The listing builds one solid part. Answer for the finished solid, in the listing's coordinates (mm). Face numbers are marked on the shaded views. A direction names the side the tool comes from. Round coordinates to 2 decimals unless told otherwise and drop trailing zeros. Write each loop counter-clockwise with the first axis right and the second up, starting at its lowest first coordinate (ties: lowest second). Pieces come first, ordered by that corner, then holes.
Item 1: A tool of negligible diameter and unlimited length cuts with its end or side. For the marked faces 4 and 5, from which of +Z, -Z, +X, -X, +Y, -Y can it reach the whole face along a straight path? Write none if from no direction.
Item 2: Each of these flat-tipped pins is pushed along its axis until it touches: pin 1 (6.5 mm diameter, centred on x = 2.83, z = -3.52, fed in from +Y); pin 2 (12 mm diameter, centred on x = -7.5, z = -13, fed in from +Y); pin 3 (6.5 mm diameter, centred on x = 2.5, z = -2.5, fed in from +Y). Where does it stop, or does it pass through?
Item 3: For a pull along Z with two mould halves and no side action, classify the marked faces 1, 2 and 3 as +Z half, -Z half, draft (parallel to the pull), parting line (faces both ways), or undercut.
Item 4: Find section D-D on x = -7.75. Give the vertices of the cut face in (y, z).
Item 5: Find section B-B on x = 0. Give the vertices of the cut face in (y, z).
Item 6: Find section A-A on y = -3.75. Give the vertices of the cut face in (x, z), then the cut area to 3 significant figures.
Item 7: Find section C-C on z = -6.5. Give the vertices of the cut face in (x, y).
Item 8: Find the intervals of material crossed by probe 1 along Y at (x, z) = (14.25, -10); probe 2 along Z at (x, y) = (-10.5, -12); probe 3 along X at (y, z) = (-19.5, 10), in increasing order.
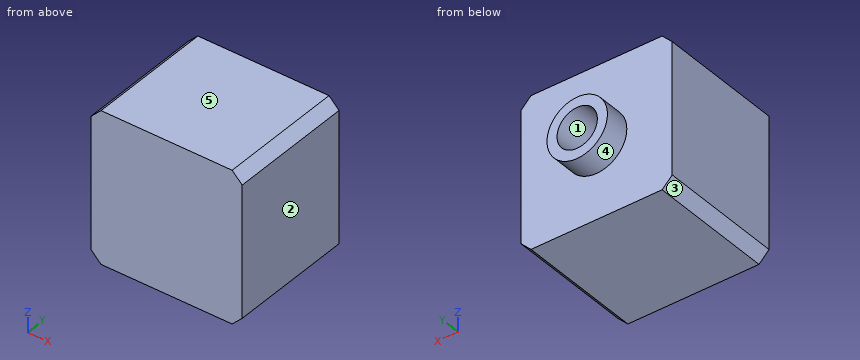
```python
from build123d import *

# Parameters (mm, degrees)
F0_W      = 30
F0_H      = 30
F1_DEPTH  = 25
F3_R      = 6
F4_DEPTH  = 5
F5_SIZE   = 2
F6_SIZE   = 2
F7_SIZE   = 2
F2_R      = 4
F8_DEPTH  = 5
F9_R      = 4
F10_DEPTH = 5


with BuildPart() as f1:
    # F0 (on Front) → F1 (new body)
    with BuildSketch(Plane.XZ):
        with Locations((2.829975, -3.521299)):
            Rectangle(F0_W, F0_H)
    extrude(amount=F1_DEPTH)

    # F3 (on face) → F4 (join)
    with BuildSketch(Plane(origin=(0, 0, 0), x_dir=(-1, 0, 0), z_dir=(0, 1, 0))):
        with Locations((-2.829975, -3.521299)):
            Circle(F3_R)
    extrude(amount=F4_DEPTH)

    # F5
    f5_edges = [f1.edges().sort_by_distance(p)[0] for p in [
        (17.829975, -12.5, 11.478701),
    ]]
    chamfer(f5_edges, length=F5_SIZE)

    # F6
    f6_edges = [f1.edges().sort_by_distance(p)[0] for p in [
        (-12.170025, -12.5, 11.478701),
    ]]
    chamfer(f6_edges, length=F6_SIZE)

    # F7
    f7_edges = [f1.edges().sort_by_distance(p)[0] for p in [
        (-12.170025, -12.5, -18.521299),
        (17.829975, -12.5, -18.521299),
    ]]
    chamfer(f7_edges, length=F7_SIZE)

    # F2 (on face) → F8 (cut)
    with BuildSketch(Plane(origin=(0, 0, 0), x_dir=(-1, 0, 0), z_dir=(0, 1, 0))):
        with Locations((-2.829975, -3.521299)):
            Circle(F2_R)
    extrude(amount=-F8_DEPTH, mode=Mode.SUBTRACT)

    # F9 (on face) → F10 (cut)
    with BuildSketch(Plane(origin=(0, 5, 0), x_dir=(-1, 0, 0), z_dir=(0, 1, 0))):
        with Locations((-2.829975, -3.521299)):
            Circle(F9_R)
    extrude(amount=-F10_DEPTH, mode=Mode.SUBTRACT)


solid = f1.part
```
Check values:
1. face 4: +Y
1. face 5: +Z, +X, -X, +Y, -Y
2. pin 1: stops at y = -5
2. pin 2: stops at y = 0
2. pin 3: stops at y = 5
3. face 1: undercut
3. face 2: draft
3. face 3: -Z half
4. outline: (-25, -18.52) - (0, -18.52) - (0, 11.48) - (-25, 11.48) - close
5. outline: (-25, -18.52) - (0, -18.52) - (0, -8.81) - (5, -8.81) - (5, -6.35) - (-5, -6.35) - (-5, -0.69) - (5, -0.69) - (5, 1.77) - (0, 1.77) - (0, 11.48) - (-25, 11.48) - close
6. outline: (-12.17, -16.52) - (-10.17, -18.52) - (15.83, -18.52) - (17.83, -16.52) - (17.83, 9.48) - (15.83, 11.48) - (-10.17, 11.48) - (-12.17, 9.48) - close; hole circle Ø8 at (2.83, -3.52)
6. area: 842 mm2
7. outline: (-12.17, -25) - (17.83, -25) - (17.83, 0) - (8.04, 0) - (8.04, 5) - (5.5, 5) - (5.5, -5) - (0.16, -5) - (0.16, 5) - (-2.38, 5) - (-2.38, 0) - (-12.17, 0) - close
8. probe 1: y = -25 to 0
8. probe 2: z = -18.19 to 11.15
8. probe 3: x = -11.65 to 17.31
